from build123d import *

# Parameters (mm, degrees)
CYLINDER128_R                   = 6
CYLINDER128_DEPTH               = 10
BOX001027045018_W               = 21
BOX001027045018_H               = 13
BOX001027045018_DEPTH           = 30
BOX001027045018_ROLL_ANGLE      = 40
BOX001027045019_W               = 21
BOX001027045019_H               = 13
BOX001027045019_DEPTH           = 30
BOX001027045019_ROLL_ANGLE      = 39.99997
BOX001027045019_PLACEMENT_ANGLE = 180
BOX001027045021_W               = 21
BOX001027045021_H               = 13
BOX001027045021_DEPTH           = 30
BOX001027045021_ROLL_ANGLE      = 40
BOX001027045021_PLACEMENT_ANGLE = 180
BOX001027045022_W               = 21
BOX001027045022_H               = 13
BOX001027045022_DEPTH           = 30
BOX001027045022_ROLL_ANGLE      = 40
BOX001027045024_W               = 21
BOX001027045024_H               = 13
BOX001027045024_DEPTH           = 30
BOX001027045024_ROLL_ANGLE      = 40
BOX001027045020_W               = 21
BOX001027045020_H               = 39
BOX001027045020_DEPTH           = 30
BOX001027045020_ROLL_ANGLE      = 39.99997
BOX001027045020_PLACEMENT_ANGLE = 180
BOX001027045017_W               = 16
BOX001027045017_H               = 32
BOX001027045017_DEPTH           = 90
CYLINDER129_R                   = 5
CYLINDER129_DEPTH               = 21


with BuildPart() as cylinder186:
    # Cylinder128 → Cylinder128 (new body)
    with BuildSketch(Plane(origin=(-5, 9, -11), x_dir=(1, 0, 0), z_dir=(0, 0, 1))):
        Circle(CYLINDER128_R)
    extrude(amount=CYLINDER128_DEPTH)


with BuildPart() as cube071:
    # Box001027045018 → Box001027045018 (new body)
    with BuildSketch(Plane.XY):
        with Locations((10.5, 6.5)):
            Rectangle(BOX001027045018_W, BOX001027045018_H)
    extrude(amount=BOX001027045018_DEPTH)


with BuildPart() as cube071_1:
    # Box001027045018 roll: moved
    add(cube071.part.rotate(Axis((0, 0, 0), (1, 0, 0)), BOX001027045018_ROLL_ANGLE))


with BuildPart() as cube071_2:
    # Box001027045018 placement: moved
    add(cube071_1.part.moved(Location((-11, -16.5, 27.4))))


with BuildPart() as cube072:
    # Box001027045019 → Box001027045019 (new body)
    with BuildSketch(Plane.XY):
        with Locations((10.5, 6.5)):
            Rectangle(BOX001027045019_W, BOX001027045019_H)
    extrude(amount=BOX001027045019_DEPTH)


with BuildPart() as cube072_1:
    # Box001027045019 roll: moved
    add(cube072.part.rotate(Axis((0, 0, 0), (1, 0, 0)), BOX001027045019_ROLL_ANGLE))


with BuildPart() as cube072_2:
    # Box001027045019 placement: moved
    add(cube072_1.part.moved(Location((11, 16.5, 38.4))).rotate(Axis((11, 16.5, 38.4), (0, 0, 1)), BOX001027045019_PLACEMENT_ANGLE))


with BuildPart() as cube074:
    # Box001027045021 → Box001027045021 (new body)
    with BuildSketch(Plane.XY):
        with Locations((10.5, 6.5)):
            Rectangle(BOX001027045021_W, BOX001027045021_H)
    extrude(amount=BOX001027045021_DEPTH)


with BuildPart() as cube074_1:
    # Box001027045021 roll: moved
    add(cube074.part.rotate(Axis((0, 0, 0), (1, 0, 0)), BOX001027045021_ROLL_ANGLE))


with BuildPart() as cube074_2:
    # Box001027045021 placement: moved
    add(cube074_1.part.moved(Location((11, 16.5, 16.4))).rotate(Axis((11, 16.5, 16.4), (0, 0, 1)), BOX001027045021_PLACEMENT_ANGLE))


with BuildPart() as cube075:
    # Box001027045022 → Box001027045022 (new body)
    with BuildSketch(Plane.XY):
        with Locations((10.5, 6.5)):
            Rectangle(BOX001027045022_W, BOX001027045022_H)
    extrude(amount=BOX001027045022_DEPTH)


with BuildPart() as cube075_1:
    # Box001027045022 roll: moved
    add(cube075.part.rotate(Axis((0, 0, 0), (1, 0, 0)), BOX001027045022_ROLL_ANGLE))


with BuildPart() as cube075_2:
    # Box001027045022 placement: moved
    add(cube075_1.part.moved(Location((-11, -16.5, 49.4))))


with BuildPart() as cube077:
    # Box001027045024 → Box001027045024 (new body)
    with BuildSketch(Plane.XY):
        with Locations((10.5, 6.5)):
            Rectangle(BOX001027045024_W, BOX001027045024_H)
    extrude(amount=BOX001027045024_DEPTH)


with BuildPart() as cube077_1:
    # Box001027045024 roll: moved
    add(cube077.part.rotate(Axis((0, 0, 0), (1, 0, 0)), BOX001027045024_ROLL_ANGLE))


with BuildPart() as cube077_2:
    # Box001027045024 placement: moved
    add(cube077_1.part.moved(Location((-11, -16.5, 71.4))))


with BuildPart() as fusion112034:
    # Box001027045020 → Box001027045020 (new body)
    with BuildSketch(Plane.XY):
        with Locations((10.5, 19.5)):
            Rectangle(BOX001027045020_W, BOX001027045020_H)
    extrude(amount=BOX001027045020_DEPTH)


with BuildPart() as fusion112034_1:
    # Box001027045020 roll: moved
    add(fusion112034.part.rotate(Axis((0, 0, 0), (1, 0, 0)), BOX001027045020_ROLL_ANGLE))


with BuildPart() as fusion112034_2:
    # Box001027045020 placement: moved
    add(fusion112034_1.part.moved(Location((11, 16.5, 60.4))).rotate(Axis((11, 16.5, 60.4), (0, 0, 1)), BOX001027045020_PLACEMENT_ANGLE))

    # Fusion112034: union Cube071, Cube072, Cube074, Cube075, Cube077
    add(cube071_2.part)
    add(cube072_2.part)
    add(cube074_2.part)
    add(cube075_2.part)
    add(cube077_2.part)


with BuildPart() as fusion112035:
    # Box001027045017 → Box001027045017 (new body)
    with BuildSketch(Plane(origin=(-8, -16, -11), x_dir=(1, 0, 0), z_dir=(0, 0, 1))):
        with Locations((8, 16)):
            Rectangle(BOX001027045017_W, BOX001027045017_H)
    extrude(amount=BOX001027045017_DEPTH)

    # Cut070: cut Fusion112034
    add(fusion112034_2.part, mode=Mode.SUBTRACT)

    # Fusion112035: union Cylinder186
    add(cylinder186.part)


with BuildPart() as body_blank:
    # Cylinder129 → Cylinder129 (new body)
    with BuildSketch(Plane(origin=(0, 13, -11), x_dir=(1, 0, 0), z_dir=(0, 0, 1))):
        Circle(CYLINDER129_R)
    extrude(amount=CYLINDER129_DEPTH)

    # Fusion112036: union Fusion112035
    add(fusion112035.part)


solid = body_blank.part
Input: part model. Units: mm. Frame: model coordinates. A direction names the side the tool comes from. Give positions to 0.01 mm unless a question says otherwise; leave off trailing zeros. Write each loop counter-clockwise with the first axis right and the second up, starting at its lowest first coordinate (ties: lowest second). Pieces come first, ordered by that corner, then holes.
Q1. Section C-C, the plane y = -12. Output: boundary loops of the cut face in (x, z).
Q2. Pull-direction query (Z, two-part tool) for faces 1 (the face through (-5, 16, 6)), 2 (the face through (-0.112, -11.205, 53.843)), 3 (the face through (-2, 1, -11)); classes: pulls with the +Z half, pulls with the -Z half, needs draft (parallel to the pull), parting line crosses it, or undercut.
Q3. Set-up query: faces 4 (the face through (8, 0, 33)), 5 (the face through (0.112, 11.204, 42.843)), 6 (the face through (-0.112, -11.205, 31.843)), 7 (the face through (0, 17, 10)). Return all of +Z, -Z, +X, -X, +Y, -Y with unobstructed straight access to the full face (end or side cutting, diameter ignored); none if empty.
Q4. Section D-D, the plane x = -3. Output: boundary loops of the cut face in (y, z).
Q5. Section A-A, the plane z = -2. Output: boundary loops of the cut face in (x, y), plus the area to 3 significant figures.
Q6. Section B-B, the plane x = -6.5. Output: boundary loops of the cut face in (y, z), plus the area to 3 significant figures.
Q7. Material intervals for probe 1 along Z at (x, y) = (-6.5, -13.5); probe 2 along Z at (x, y) = (1.25, 14); probe 3 along X at (y, z) = (4, 5), sorted ascending.
Q8. First-contact query: P1, Ø4, axis at x = -2, y = -10.5, coming from the +Z side; P2, Ø10, axis at y = -10.5, z = 32.5, coming from the -X side; P3, Ø1, axis at x = -8, z = 59, coming from the -Y side; P4, Ø1.5, axis at y = 13.5, z = 53, coming from the +X side. Flat tips, straight axial feed; report the tip coordinate or a pass-through.
Filled in:
1. outline: (-8, -11) - (8, -11) - (8, 31.18) - (-8, 31.18) - close; (-8, 42.26) - (8, 42.26) - (8, 53.18) - (-8, 53.18) - close; (-8, 64.26) - (8, 64.26) - (8, 75.18) - (-8, 75.18) - close
2. face 1: needs draft
2. face 2: undercut
2. face 3: pulls with the -Z half
3. face 4: +Z, -Z, +X, +Y, -Y
3. face 5: +X, -X, +Y
3. face 6: +X, -X, -Y
3. face 7: +Z, +X, -X, +Y
4. outline: (-16, -11) - (17, -11) - (17, 10) - (16, 10) - (16, 16.82) - (6.54, 24.76) - (16, 36.03) - (16, 38.82) - (6.54, 46.76) - (16, 58.03) - (16, 60.82) - (-5.67, 79) - (-7.44, 79) - (-16, 71.82) - (-16, 69.03) - (-6.54, 57.76) - (-16, 49.82) - (-16, 47.03) - (-6.54, 35.76) - (-16, 27.82) - close
5. outline: (-8, -16) - (8, -16) - (8, 16) - (4, 16) arc R5 ccw to (-4, 16) - (-8, 16) - (-8, 14.2) arc R6 ccw to (-8, 3.8) - close
5. area: 545 mm2
6. outline: (-16, -11) - (16, -11) - (16, 16.82) - (6.54, 24.76) - (16, 36.03) - (16, 38.82) - (6.54, 46.76) - (16, 58.03) - (16, 60.82) - (-5.67, 79) - (-7.44, 79) - (-16, 71.82) - (-16, 69.03) - (-6.54, 57.76) - (-16, 49.82) - (-16, 47.03) - (-6.54, 35.76) - (-16, 27.82) - close
6. area: 2,290 mm2
7. probe 1: z = -11 to 29.92, 44.05 to 51.92, 66.05 to 73.92
7. probe 2: z = -11 to 18.5, 33.65 to 40.5, 55.65 to 62.5
7. probe 3: x = -8 to 8
8. P1: stops at z = 78.11
8. P2: stops at x = -8
8. P3: stops at y = -8
8. P4: passes through
